Verification items for the finished model (mm, model axes). Face numbers are marked on the shaded views. A direction names the side the tool comes from. Coordinates: 2 decimals unless noted, no trailing zeros. Loops run counter-clockwise (first coordinate to the right, second up) from the corner with the lowest first, then second, coordinate; pieces in that order, holes last. Notation, with made-up numbers: (-9.5, -28) - (46.5, -28) arc R23 ccw to (46.5, -10) - close; hole circle Ø10 at (65.25, -33). An arc over 180 degrees is marked (long way). Answer as CSV lines item,"result". Start each with the question number.
1. Cross-section at A-A (x = 15.5). Enter the section's corners in (y, z), plus the area to 3 significant figures.
2. Release check for a two-part mould opening along X. For the marked faces 1, 2, 3 and 4 record: pulls with the +X half, pulls with the -X half, needs draft (parallel to the pull), parting line crosses it, or undercut.
3. Cross-section at C-C (y = 2.8). Enter the section's corners in (x, z), plus the area to 3 significant figures.
4. Cross-section at D-D (x = -2). Enter the section's corners in (y, z).
5. Cross-section at B-B (z = -16). Enter the section's corners in (x, y), plus the area to 3 significant figures.
6. Material ranges on line 1 (X direction, y = 4.1, z = 0.5); line 2 (X direction, y = 2.75, z = -15.5); line 3 (Z direction, x = 16, y = 3.55), recorded low to high. Write a range as [from, to].
7. Gauge pin test, flat ends, axial feed: P1, Ø3, axis at x = -1, y = 1.5, coming from the +Z side; P2, Ø1.5, axis at x = 0, y = 1.5, coming from the -Z side; P3, Ø2.5, axis at y = 3, z = 1, coming from the +X side. Record the tip position at first contact, or that the pin passes through.
8. Set-up check for the marked faces 5 and 6: record each of +Z, -Z, +X, -X, +Y, -Y from which the full face is reachable in a straight line by a thin tool's end or side.
```python
from build123d import *

# Parameters (mm, degrees)
SKETCH_1_W      = 42
SKETCH_1_H      = 42
SKETCH_1_R      = 11.05
SKETCH_1_R_2    = 1.75
EXTRUDE_1_DEPTH = 5
EXTRUDE_2_DEPTH = 5


with BuildPart() as part:
    # 草图1 → 凸台-拉伸1 (new body)
    with BuildSketch(Plane(origin=(0, 0, 0), x_dir=(1, 0, 0), z_dir=(0, 1, 0))):
        Rectangle(SKETCH_1_W, SKETCH_1_H)
        with Locations(Location((0, 0, 0), (0, 0, 270))):
            Circle(SKETCH_1_R, mode=Mode.SUBTRACT)
        with Locations(Location((15.5, 15.5, 0), (0, 0, 270))):
            Circle(SKETCH_1_R_2, mode=Mode.SUBTRACT)
        with Locations(Location((15.5, -15.5, 0), (0, 0, 270))):
            Circle(SKETCH_1_R_2, mode=Mode.SUBTRACT)
        with Locations(Location((-15.5, -15.5, 0), (0, 0, 270))):
            Circle(SKETCH_1_R_2, mode=Mode.SUBTRACT)
        with Locations(Location((-15.5, 15.5, 0), (0, 0, 270))):
            Circle(SKETCH_1_R_2, mode=Mode.SUBTRACT)
    extrude(amount=EXTRUDE_1_DEPTH)

    # 草图2 → 凸台-拉伸2 (add)
    with BuildSketch(Plane(origin=(0, 0, 0), x_dir=(1, 0, 0), z_dir=(0, 1, 0))):
        with BuildLine():
            Line((-5.80218169, -21), (-21, -21))
            Line((-21, -21), (-21, -5.80218169))
            ThreePointArc((-21, -5.80218169), (-22.086185579, -11.829035113), (-25.208061098, -17.097493573))
            ThreePointArc((-25.208061098, -17.097493573), (-24.925514037, -24.925514037), (-17.097493573, -25.208061098))
            ThreePointArc((-17.097493573, -25.208061098), (-11.829035113, -22.086185579), (-5.80218169, -21))
        make_face()
        with BuildLine():
            Line((21, -5.80218169), (21, -21))
            Line((21, -21), (5.80218169, -21))
            ThreePointArc((5.80218169, -21), (11.829035113, -22.086185579), (17.097493573, -25.208061098))
            ThreePointArc((17.097493573, -25.208061098), (24.925514037, -24.925514037), (25.208061098, -17.097493573))
            ThreePointArc((25.208061098, -17.097493573), (22.086185579, -11.829035113), (21, -5.80218169))
        make_face()
        with BuildLine():
            Line((-21, 5.80218169), (-21, 21))
            Line((-21, 21), (-5.80218169, 21))
            ThreePointArc((-5.80218169, 21), (-11.829035113, 22.086185579), (-17.097493573, 25.208061098))
            ThreePointArc((-17.097493573, 25.208061098), (-24.925514037, 24.925514037), (-25.208061098, 17.097493573))
            ThreePointArc((-25.208061098, 17.097493573), (-22.086185579, 11.829035113), (-21, 5.80218169))
        make_face()
        with BuildLine():
            Line((5.80218169, 21), (21, 21))
            Line((21, 21), (21, 5.80218169))
            ThreePointArc((21, 5.80218169), (22.086185579, 11.829035113), (25.208061098, 17.097493573))
            ThreePointArc((25.208061098, 17.097493573), (24.925514037, 24.925514037), (17.097493573, 25.208061098))
            ThreePointArc((17.097493573, 25.208061098), (11.829035113, 22.086185579), (5.80218169, 21))
        make_face()
    extrude(amount=EXTRUDE_2_DEPTH)


solid = part.part
```
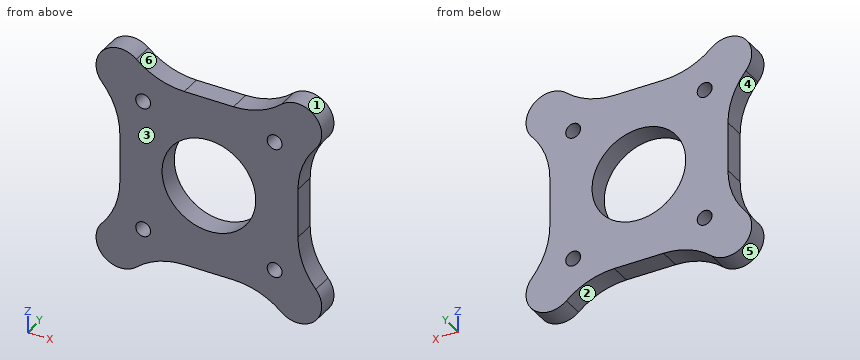
Values follow:
1,outline,"(0, -23.98) - (5, -23.98) - (5, -17.25) - (0, -17.25) - close; (0, -13.75) - (5, -13.75) - (5, 13.75) - (0, 13.75) - close; (0, 17.25) - (5, 17.25) - (5, 23.98) - (0, 23.98) - close"
1,area,"205 mm²"
2,face 1,"undercut"
2,face 2,"undercut"
2,face 3,"needs draft"
2,face 4,"pulls with the -X half"
3,outline,"(-25.21, -17.1) arc R5.75 ccw to (-17.1, -25.21) arc R17.26 cw to (-5.8, -21) - (5.8, -21) arc R17.26 cw to (17.1, -25.21) arc R5.75 ccw to (25.21, -17.1) arc R17.26 cw to (21, -5.8) - (21, 5.8) arc R17.26 cw to (25.21, 17.1) arc R5.75 ccw to (17.1, 25.21) arc R17.26 cw to (5.8, 21) - (-5.8, 21) arc R17.26 cw to (-17.1, 25.21) arc R5.75 ccw to (-25.21, 17.1) arc R17.26 cw to (-21, 5.8) - (-21, -5.8) arc R17.26 cw to start; hole circle Ø3.5 at (-15.5, -15.5); hole circle Ø3.5 at (-15.5, 15.5); hole circle Ø22.1 at (0, 0); hole circle Ø3.5 at (15.5, -15.5); hole circle Ø3.5 at (15.5, 15.5)"
3,area,"1,720 mm²"
4,outline,"(0, -21) - (5, -21) - (5, -10.87) - (0, -10.87) - close; (0, 10.87) - (5, 10.87) - (5, 21) - (0, 21) - close"
5,outline,"(-24.33, 0) - (-17.18, 0) - (-17.18, 5) - (-24.33, 5) - close; (-13.82, 0) - (13.82, 0) - (13.82, 5) - (-13.82, 5) - close; (17.18, 0) - (24.33, 0) - (24.33, 5) - (17.18, 5) - close"
5,area,"210 mm²"
6,line 1,"x = [-21, -11.04], [11.04, 21]"
6,line 2,"x = [-23.98, -17.25], [-13.75, 13.75], [17.25, 23.98]"
6,line 3,"z = [-24.33, -17.18], [-13.82, 13.82], [17.18, 24.33]"
7,P1,"stops at z = 21"
7,P2,"stops at z = -21"
7,P3,"stops at x = 21"
8,face 5,"+Y, -Y"
8,face 6,"+Z, +Y, -Y"
